Build history of the part. All positions in model axes, mm. Face numbers are marked on the shaded views. A direction names the side the tool comes from. Coordinates: 2 decimals unless noted, no trailing zeros. Loops run counter-clockwise (first coordinate to the right, second up) from the corner with the lowest first, then second, coordinate; pieces in that order, holes last.
(1) Slice it at A-A (z = 8). Give the cut face in (x, y).
(2) Wall check: L1, parallel to Y at x = 0, z = 2.45; L2, parallel to Z at x = 7.5, y = -2.5; L3, parallel to Z at x = -0.75, y = 0. Give the ranges that are in metal, low to high.
(3) Slice it at C-C (z = 13.5). Give the cut face in (x, y), and give its area (4 significant figures).
(4) Slice it at B-B (z = 32.5). Give the cut face in (x, y), and give its area (3 significant figures).
(5) Tool access for the marked faces 1, 2, 3, 4 and 5: list every direction of +Z, -Z, +X, -X, +Y, -Y with a clear straight run to the whole face (end or side of a thin tool).
(6) Two-plate mould, pull along Y, no slides. Class the marked faces 6, 7 and 8: pulls with the +Y half, pulls with the -Y half, needs draft (parallel to the pull), parting line crosses it, or undercut.
(7) Flat gauge pins, fed straight in: P1, Ø0.6, axis at y = -6, z = 7.5, coming from the +X side; P2, Ø2.5, axis at x = 6.5, z = 4.5, coming from the -Y side; P3, Ø1.7, axis at x = 7, y = -0.5, coming from the +Z side. Where does each tip first touch, or does it go through?
from build123d import *

# Parameters (mm, degrees)
BOX001_W          = 2
BOX001_H          = 2.5
BOX001_DEPTH      = 2.5
ARRAY001_COUNT    = 4
CYLINDER003_R     = 4.6
CYLINDER003_DEPTH = 2.5
BOX002_W          = 6.5
BOX002_H          = 6.5
BOX002_DEPTH      = 5
CYLINDER004_R     = 3.2
CYLINDER004_DEPTH = 18.5
CYLINDER001_W     = 9
CYLINDER001_H     = 6
CYLINDER001_ANGLE = 90
ARRAY_COUNT       = 4
CYLINDER006_R     = 4.5
CYLINDER006_DEPTH = 2
CYLINDER007_R     = 2.5
CYLINDER007_DEPTH = 6
CYLINDER_R        = 9
CYLINDER_DEPTH    = 2.65
FILLET_R          = 1
FILLET001_R       = 1
FILLET002_R       = 1
FILLET003_R       = 1
CYLINDER005_R     = 2
CYLINDER005_DEPTH = 5
FILLET004_R       = 1
BOX_W             = 9.2
BOX_H             = 9.2
BOX_DEPTH         = 2.5


with BuildPart() as array001:
    # Box001 → Box001 (new body)
    with BuildSketch(Plane(origin=(4.6, -1.25, 6), x_dir=(1, 0, 0), z_dir=(0, 0, 1))):
        with Locations((1, 1.25)):
            Rectangle(BOX001_W, BOX001_H)
    extrude(amount=BOX001_DEPTH)

    # Array001: Array001 ×4 about axis
    array001_axis = Axis((0, 0, 0), (0, 0, 1))


with BuildPart() as array001_1:
    add(array001.part)
    for i in range(1, ARRAY001_COUNT):
        add(array001.part.rotate(array001_axis, i * 360 / ARRAY001_COUNT))


with BuildPart() as cilindro003:
    # Cylinder003 → Cylinder003 (new body)
    with BuildSketch(Plane.XY.offset(8.5)):
        Circle(CYLINDER003_R)
    extrude(amount=CYLINDER003_DEPTH)


with BuildPart() as cubo002:
    # Box002 → Box002 (new body)
    with BuildSketch(Plane(origin=(-3.25, -3.25, 11), x_dir=(1, 0, 0), z_dir=(0, 0, 1))):
        with Locations((3.25, 3.25)):
            Rectangle(BOX002_W, BOX002_H)
    extrude(amount=BOX002_DEPTH)


with BuildPart() as cilindro004:
    # Cylinder004 → Cylinder004 (new body)
    with BuildSketch(Plane.XY.offset(16)):
        Circle(CYLINDER004_R)
    extrude(amount=CYLINDER004_DEPTH)


with BuildPart() as array:
    # Cylinder001 → Cylinder001 (revolve)
    with BuildSketch(Plane(origin=(4.6, 4.6, 0), x_dir=(1, 0, 0), z_dir=(0, -1, 0))):
        with Locations((4.5, 3)):
            Rectangle(CYLINDER001_W, CYLINDER001_H)
    revolve(axis=Axis((4.6, 4.6, 0), (0, 0, 1)), revolution_arc=CYLINDER001_ANGLE)

    # Array: Array ×4 about axis
    array_axis = Axis((0, 0, 0), (0, 0, 1))


with BuildPart() as array_1:
    add(array.part)
    for i in range(1, ARRAY_COUNT):
        add(array.part.rotate(array_axis, i * 360 / ARRAY_COUNT))


with BuildPart() as cilindro006:
    # Cylinder006 → Cylinder006 (new body)
    with BuildSketch(Plane.XY.offset(2)):
        Circle(CYLINDER006_R)
    extrude(amount=CYLINDER006_DEPTH)


with BuildPart() as cilindro007:
    # Cylinder007 → Cylinder007 (new body)
    with BuildSketch(Plane.XY.offset(4)):
        Circle(CYLINDER007_R)
    extrude(amount=CYLINDER007_DEPTH)


with BuildPart() as cut001:
    # Cylinder → Cylinder (new body)
    with BuildSketch(Plane.XY.offset(2)):
        Circle(CYLINDER_R)
    extrude(amount=CYLINDER_DEPTH)

    # Cut: cut Cilindro007
    add(cilindro007.part, mode=Mode.SUBTRACT)

    # Cut001: cut Cilindro006
    add(cilindro006.part, mode=Mode.SUBTRACT)


with BuildPart() as fillet003:
    # Cone → Cone (revolve)
    with BuildSketch(Plane(origin=(0, 0, 4.5), x_dir=(1, 0, 0), z_dir=(0, -1, 0))):
        Polygon((0, 0), (7.5, 0), (6.75, 1.5), (0, 1.5), align=None)
    revolve(axis=Axis((0, 0, 4.5), (0, 0, 1)))

    # Fusion: union Cut001
    add(cut001.part)

    # Cut002: cut Array
    add(array_1.part, mode=Mode.SUBTRACT)

    # Fillet
    fillet_edges = [fillet003.edges().sort_by_distance(p)[0] for p in [
        (0, 9, 4.65),
    ]]
    fillet(fillet_edges, radius=FILLET_R)

    # Fillet001
    fillet001_edges = [fillet003.edges().sort_by_distance(p)[0] for p in [
        (-9, 0, 4.65),
    ]]
    fillet(fillet001_edges, radius=FILLET001_R)

    # Fillet002
    fillet002_edges = [fillet003.edges().sort_by_distance(p)[0] for p in [
        (0, -9, 4.65),
    ]]
    fillet(fillet002_edges, radius=FILLET002_R)

    # Fillet003
    fillet003_edges = [fillet003.edges().sort_by_distance(p)[0] for p in [
        (8.678153, 2.3853, 4.65),
    ]]
    fillet(fillet003_edges, radius=FILLET003_R)


with BuildPart() as fillet004:
    # Cylinder005 → Cylinder005 (new body)
    with BuildSketch(Plane.XY.offset(34)):
        Circle(CYLINDER005_R)
    extrude(amount=CYLINDER005_DEPTH)

    # Fillet004
    fillet004_edges = [fillet004.edges().sort_by_distance(p)[0] for p in [
        (-2, 0, 39),
    ]]
    fillet(fillet004_edges, radius=FILLET004_R)


with BuildPart() as fusion001:
    # Box → Box (new body)
    with BuildSketch(Plane(origin=(-4.6, -4.6, 6), x_dir=(1, 0, 0), z_dir=(0, 0, 1))):
        with Locations((4.6, 4.6)):
            Rectangle(BOX_W, BOX_H)
    extrude(amount=BOX_DEPTH)

    # Fusion001: union Array001, Cilindro003, Cubo002, Cilindro004, Fillet003, Fillet004
    add(array001_1.part)
    add(cilindro003.part)
    add(cubo002.part)
    add(cilindro004.part)
    add(fillet003.part)
    add(fillet004.part)


solid = fusion001.part
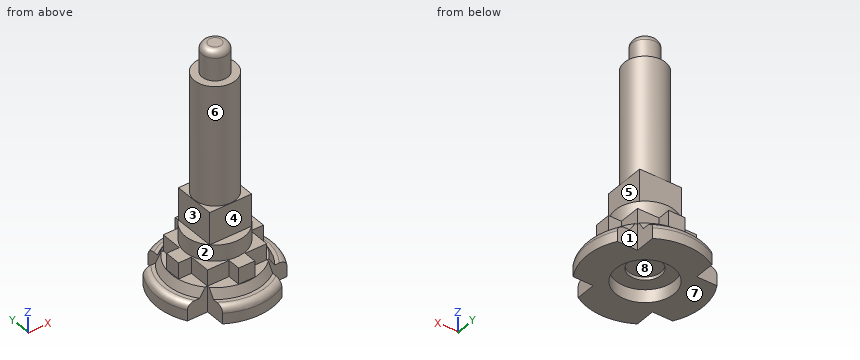
Response values:
1. outline: (-6.6, -1.25) - (-4.6, -1.25) - (-4.6, -4.6) - (-1.25, -4.6) - (-1.25, -6.6) - (1.25, -6.6) - (1.25, -4.6) - (4.6, -4.6) - (4.6, -1.25) - (6.6, -1.25) - (6.6, 1.25) - (4.6, 1.25) - (4.6, 4.6) - (1.25, 4.6) - (1.25, 6.6) - (-1.25, 6.6) - (-1.25, 4.6) - (-4.6, 4.6) - (-4.6, 1.25) - (-6.6, 1.25) - close
2. L1: y = -9 to -4.5, 4.5 to 9
2. L2: z = 2 to 4.65
2. L3: z = 4.5 to 39
3. outline: (-3.25, -3.25) - (3.25, -3.25) - (3.25, 3.25) - (-3.25, 3.25) - close
3. area: 42.25 mm2
4. outline: circle Ø6.4 at (0, 0)
4. area: 32.2 mm2
5. face 1: +Z, -Z, +X, +Y
5. face 2: +Z
5. face 3: +Z, -X, +Y, -Y
5. face 4: +Z, +X, -X, -Y
5. face 5: +Z, +X, +Y, -Y
6. face 6: parting line crosses it
6. face 7: needs draft
6. face 8: undercut
7. P1: stops at x = 1.25
7. P2: stops at y = -4.6
7. P3: stops at z = 8.5
